```python
from build123d import *

# Parameters (mm, degrees)
SKETCH1_R           = 1.25
SKETCH1_R_2         = 1.35
SKETCH1_R_3         = 4.675
BOSS_EXTRUDE2_DEPTH = 4
SKETCH2_R           = 2.75
CUT_EXTRUDE1_DEPTH  = 1
SKETCH4_R           = 3
SKETCH4_R_2         = 1.35
BOSS_EXTRUDE3_DEPTH = 2.45


with BuildPart() as part:
    # Sketch1 → Boss-Extrude2 (new body)
    with BuildSketch(Plane(origin=(0, 0, 0), x_dir=(1, 0, 0), z_dir=(0, 1, 0))):
        with BuildLine():
            ThreePointArc((6.823529412, -9.705882353), (23, 0), (6.823529412, 9.705882353))
            ThreePointArc((6.823529412, 9.705882353), (-2.298574999, 6.194299994), (-12, 5))
            ThreePointArc((-12, 5), (-17, 0), (-12, -5))
            ThreePointArc((-12, -5), (-2.298574999, -6.194299994), (6.823529412, -9.705882353))
        make_face()
        with Locations(Location((4.2, 0, 0), (0, 0, 270))):
            Circle(SKETCH1_R, mode=Mode.SUBTRACT)
        with Locations(Location((-12, 0, 0), (0, 0, 270))):
            Circle(SKETCH1_R_2, mode=Mode.SUBTRACT)
        with Locations(Location((12, 7.8, 0), (0, 0, 270))):
            Circle(SKETCH1_R, mode=Mode.SUBTRACT)
        with Locations(Location((19.8, 0, 0), (0, 0, 270))):
            Circle(SKETCH1_R, mode=Mode.SUBTRACT)
        with Locations(Location((12, -7.8, 0), (0, 0, 270))):
            Circle(SKETCH1_R, mode=Mode.SUBTRACT)
        with Locations(Location((12, 0, 0), (0, 0, 270))):
            Circle(SKETCH1_R_3, mode=Mode.SUBTRACT)
    extrude(amount=BOSS_EXTRUDE2_DEPTH)

    # Sketch2 → Cut-Extrude1 (cut)
    with BuildSketch(Plane.XZ):
        with Locations(Location((12, -7.8, 0), (0, 0, 270))):
            Circle(SKETCH2_R)
        with Locations(Location((4.2, 0, 0), (0, 0, 270))):
            Circle(SKETCH2_R)
        with Locations(Location((12, 7.8, 0), (0, 0, 270))):
            Circle(SKETCH2_R)
        with Locations(Location((19.8, 0, 0), (0, 0, 270))):
            Circle(SKETCH2_R)
    extrude(amount=-CUT_EXTRUDE1_DEPTH, mode=Mode.SUBTRACT)

    # Sketch4 → Boss-Extrude3 (add)
    with BuildSketch(Plane(origin=(0, 4, 0), x_dir=(1, 0, 0), z_dir=(0, 1, 0))):
        with Locations(Location((-12, 0, 0), (0, 0, 270))):
            Circle(SKETCH4_R)
        with Locations(Location((-12, 0, 0), (0, 0, 270))):
            Circle(SKETCH4_R_2, mode=Mode.SUBTRACT)
    extrude(amount=BOSS_EXTRUDE3_DEPTH)


solid = part.part
```
Geometry: final body of the model. Coordinates: model frame, mm. A direction names the side the tool comes from. Coordinates: 2 decimals unless noted, no trailing zeros. Write each loop counter-clockwise with the first axis right and the second up, starting at its lowest first coordinate (ties: lowest second). Pieces come first, ordered by that corner, then holes. Notation, with made-up numbers: M 12,24.25 L 42,24.25 A18 ccw 42,52.25 Z; hole C 13.5,25 d9. An arc over 180 degrees is marked long. Answer as CSV lines item,"result". Start each with the question number.
Q1. Line query: line 1 (X direction, y = 3.25, z = -0.25); line 2 (Y direction, x = 9.5, z = 6.25); line 3 (Z direction, x = 4.2, y = 1.85). Output: solid intervals per line, ascending. Write a range as from..to.
Q2. Cut plane C-C on x = 19.8. Return the cut outline in (y, z), then the cut area to 3 significant figures.
Q3. Reachability of faces 1 (the flat face through (11, 1, -9)), 2 (the cylindrical face through (-17, 2, 0)) from +Z, -Z, +X, -X, +Y, -Y: full face, straight path, thin tool, end or side. Return the list, or none.
Q4. Cut plane B-B on y = 1.5. Return the cut outline in (x, z) (3 decimals), then the cut area to 3 significant figures.
Q5. Cut plane D-D on z = -7.8. Return the cut outline in (x, y), then the cut area to 3 significant figures.
Q6. Mould query, pull axis Z, two halves, no side actions, for faces 3 (the cylindrical face through (5.44, 2.48, -0.16)), 4 (the flat face through (3, 0, -3)), 5 (the cylindrical face through (-2.43, 1.97, 6.16)). Classes: released by +Z, released by -Z, zero draft, split by the parting line, or undercut.
Q7. Cut plane A-A on x = 12. Return the cut outline in (y, z) (3 decimals).
Q8. Pin query (flat end, axial travel): P1, Ø3.5, axis at x = 12, z = -7.8, coming from the +Y side; P2, Ø3, axis at y = 4.5, z = -5.5, coming from the +X side; P3, Ø3, axis at x = 12, z = 7.8, coming from the -Y side; P4, Ø2, axis at x = 5.5, z = -6.5, coming from the -Y side. Return the tip coordinate at first contact, or that it passes through.
Findings below:
1,line 1,"x = -16.99..-13.33, -10.67..2.98, 5.42..7.33, 16.67..18.58, 21.02..23"
1,line 2,"y = 0..4"
1,line 3,"z = -8.43..-1.25, 1.25..8.43"
2,outline,"M 0,-7.76 L 4,-7.76 L 4,-1.25 L 1,-1.25 L 1,-2.75 L 0,-2.75 Z; M 0,2.75 L 1,2.75 L 1,1.25 L 4,1.25 L 4,7.76 L 0,7.76 Z"
2,area,"49.1 mm2"
3,face 1,"-Y"
3,face 2,"-X, +Y, -Y"
4,outline,"M -12,-5 A40 cw 6.824,-9.706 A11 ccw long 6.824,9.706 A40 cw -12,5 A5 ccw Z; hole C -12,0 d2.7; hole C 4.2,0 d2.5; hole C 12,0 d9.35; hole C 12,-7.8 d2.5; hole C 12,7.8 d2.5; hole C 19.8,0 d2.5"
4,area,"491 mm2"
5,outline,"M 2.7,0 L 9.25,0 L 9.25,1 L 10.75,1 L 10.75,4 L 2.7,4 Z; M 13.25,1 L 14.75,1 L 14.75,0 L 19.76,0 L 19.76,4 L 13.25,4 Z"
5,area,"55.2 mm2"
6,face 3,"undercut"
6,face 4,"zero draft"
6,face 5,"released by +Z"
7,outline,"M 0,-11 L 4,-11 L 4,-9.05 L 1,-9.05 L 1,-10.55 L 0,-10.55 Z; M 0,-5.05 L 1,-5.05 L 1,-6.55 L 4,-6.55 L 4,-4.675 L 0,-4.675 Z; M 0,4.675 L 4,4.675 L 4,6.55 L 1,6.55 L 1,5.05 L 0,5.05 Z; M 0,10.55 L 1,10.55 L 1,9.05 L 4,9.05 L 4,11 L 0,11 Z"
8,P1,"stops at y = 4"
8,P2,"stops at x = 22.21"
8,P3,"stops at y = 1"
8,P4,"stops at y = 0"
